from build123d import *

# Parameters (mm, degrees)
F1_DEPTH = 12.7


with BuildPart() as f1:
    # F0 (on Right) → F1 (new body, symmetric)
    with BuildSketch(Plane.YZ):
        with BuildLine():
            Line((130.597452, 0), (246.722493, 0))
            ThreePointArc((246.722493, 0), (264.683005, 7.439488), (272.122493, 25.4))
            Line((272.122493, 25.4), (272.122493, 76.2))
            ThreePointArc((272.122493, 76.2), (264.683005, 94.160512), (246.722493, 101.6))
            Line((246.722493, 101.6), (-58.077507, 101.6))
            ThreePointArc((-58.077507, 101.6), (-76.038019, 94.160512), (-83.477507, 76.2))
            Line((-83.477507, 76.2), (-83.477507, 25.4))
            ThreePointArc((-83.477507, 25.4), (-76.038019, 7.439488), (-58.077507, 0))
            Line((-58.077507, 0), (-49.55408, 0))
            ThreePointArc((-49.55408, 0), (-35.497441, -4.244128), (-26.138297, -15.558196))
            Line((-26.138297, -15.558196), (209.428738, -576.023158))
            ThreePointArc((209.428738, -576.023158), (266.624167, -600.185809), (292.175695, -543.597205))
            Line((292.175695, -543.597205), (106.72926, -34.087312))
            ThreePointArc((106.72926, -34.087312), (109.790991, -10.831159), (130.597452, 0))
        make_face()
    extrude(amount=F1_DEPTH, both=True)


solid = f1.part
Design review of the part built by this model. Coordinates are the model's own, in mm. A direction names the side the tool comes from. Round coordinates to 2 decimals unless told otherwise and drop trailing zeros. Write each loop counter-clockwise with the first axis right and the second up, starting at its lowest first coordinate (ties: lowest second). Pieces come first, ordered by that corner, then holes.
Item 1: Consider section B-B on y = 119. Give the boundary of the cut face in (x, z), and give its area (3 significant figures).
Item 2: Consider section C-C on z = -201. Give the boundary of the cut face in (x, y), and give its area (3 significant figures).
Item 3: Consider section A-A on x = -7.25. Give the boundary of the cut face in (y, z), and give its area (3 significant figures).
Item 4: Consider section D-D on y = 74. Give the boundary of the cut face in (x, z), and give its area (3 significant figures).
Item 5: Draft analysis for pull direction Z (two halves, no side actions). For faces 1 (the flat face through (0.178, 89.996, -291.867)), 2 (the cylindrical face through (0.18, 109.6, -11.11)), 3 (the flat face through (0, 96, 101.6)), 4 (the flat face through (-12.7, 103, -168)), state which applies: released by +Z, released by -Z, zero draft, split by the parting line, or undercut.
Item 6: Wall thickness on L1, parallel to Y at x = 5.25, z = 55; L2, parallel to Y at x = 11.75, z = -158; L3, parallel to Z at x = 10.75, y = -61: over which ranges is each line inside the solid? List them lowest first.
Item 7: For faces 5 (the cylindrical face through (0.18, 264.48, 7.24)), 6 (the flat face through (0, 272.122, 50)), 7 (the flat face through (12.7, 103, -168)), list the 3-axis set-ups (+Z, -Z, +X, -X, +Y, -Y) from which the entire face can be reached by the end or side of a thin tool; tool diameter is ignored.
Item 8: For pin 1 Ø7 at (x, y) = (5, -55) entering from -Z; pin 2 Ø8 at (x, y) = (-2, 182.5) entering from -Z; pin 3 Ø12.5 at (x, y) = (6, 176) entering from -Z, all flat-tipped, find the tip position at first contact; note any pin that passes through.
Check values:
1. outline: (-12.7, -360.87) - (12.7, -360.87) - (12.7, -67.8) - (-12.7, -67.8) - close; (-12.7, -2.8) - (12.7, -2.8) - (12.7, 101.6) - (-12.7, 101.6) - close
1. area: 10,100 mm2
2. outline: (-12.7, 51.8) - (12.7, 51.8) - (12.7, 167.48) - (-12.7, 167.48) - close
2. area: 2,940 mm2
3. outline: (-83.48, 25.4) arc R25.4 ccw to (-58.08, 0) - (-49.55, 0) arc R25.4 cw to (-26.14, -15.56) - (209.43, -576.02) arc R44.45 ccw to (292.18, -543.6) - (106.73, -34.09) arc R25.4 cw to (130.6, 0) - (246.72, 0) arc R25.4 ccw to (272.12, 25.4) - (272.12, 76.2) arc R25.4 ccw to (246.72, 101.6) - (-58.08, 101.6) arc R25.4 ccw to (-83.48, 76.2) - close
3. area: 101,000 mm2
4. outline: (-12.7, -253.81) - (12.7, -253.81) - (12.7, 101.6) - (-12.7, 101.6) - close
4. area: 9,030 mm2
5. face 1: released by -Z
5. face 2: undercut
5. face 3: released by +Z
5. face 4: zero draft
6. L1: y = -83.48 to 272.12
6. L2: y = 33.73 to 151.83
6. L3: z = 0.17 to 101.43
7. face 5: +X, -X, +Y
7. face 6: +Z, +X, -X, +Y
7. face 7: +Z, -Z, +X, +Y, -Y
8. pin 1: stops at z = 0
8. pin 2: stops at z = -521.47
8. pin 3: stops at z = -511.36
